from build123d import *

# Parameters (mm, degrees)
SKETCH1_R           = 1.1303
SKETCH1_W           = 3.2766
SKETCH1_H           = 18.2372
BOSS_EXTRUDE1_DEPTH = 1.5875
FILLET1_R           = 4.445
SKETCH2_W           = 81.9912
SKETCH2_H           = 2.0955
BOSS_EXTRUDE2_DEPTH = 3.175
SKETCH3_W           = 31.9024
SKETCH3_H           = 2.0955
CUT_EXTRUDE1_DEPTH  = 3.175


with BuildPart() as part:
    # Sketch1 → Boss-Extrude1 (new, symmetric)
    with BuildSketch(Plane(origin=(0, 0, 0), x_dir=(1, 0, 0), z_dir=(0, 1, 0))):
        Polygon((-38.5572, -41.9227), (-38.5572, 25.0825), (38.5572, 25.0825), (38.5572, -41.9227), (54.229, -41.9227), (54.229, 41.9227), (-54.229, 41.9227), (-54.229, -41.9227), align=None)
        with Locations(Location((-40.9956, -38.6969, 0), (0, 0, 270))):
            Circle(SKETCH1_R, mode=Mode.SUBTRACT)
        with Locations(Location((-40.9956, 22.3139, 0), (0, 0, 270))):
            Circle(SKETCH1_R, mode=Mode.SUBTRACT)
        with Locations(Location((40.9956, 22.3139, 0), (0, 0, 270))):
            Circle(SKETCH1_R, mode=Mode.SUBTRACT)
        with Locations(Location((40.9956, -38.6969, 0), (0, 0, 270))):
            Circle(SKETCH1_R, mode=Mode.SUBTRACT)
        with Locations((-50.5587, 10.0711)):
            Rectangle(SKETCH1_W, SKETCH1_H, mode=Mode.SUBTRACT)
        with Locations((-50.5587, -17.8689)):
            Rectangle(SKETCH1_W, SKETCH1_H, mode=Mode.SUBTRACT)
        with Locations((50.5587, -17.8689)):
            Rectangle(SKETCH1_W, SKETCH1_H, mode=Mode.SUBTRACT)
        with Locations((50.5587, 10.0711)):
            Rectangle(SKETCH1_W, SKETCH1_H, mode=Mode.SUBTRACT)
        Polygon((-20.5232, 36.6141), (-41.7322, 36.6141), (-41.7322, 39.8907), (-9.5758, 39.8907), (-9.5758, 37.2237), (-9.5758, 36.9697), (1.5748, 36.9697), (1.5748, 28.0289), (-20.5232, 28.0289), align=None, mode=Mode.SUBTRACT)
        Polygon((9.5758, 38.590972839), (9.5758, 39.8907), (39.5478, 39.8907), (39.5478, 37.1221), (44.5262, 37.1221), (44.5262, 30.7721), (35.7632, 30.7721), (35.7632, 36.6141), (9.5758, 36.6141), align=None, mode=Mode.SUBTRACT)
    extrude(amount=BOSS_EXTRUDE1_DEPTH, both=True)

    # Fillet1
    fillet1_edges = [part.edges().sort_by_distance(p)[0] for p in [
        (-54.229, 0, -41.9227),
        (54.229, 0, -41.9227),
        (54.229, 0, 41.9227),
        (-54.229, 0, 41.9227),
    ]]
    fillet(fillet1_edges, radius=FILLET1_R)

    # Sketch2 → Boss-Extrude2 (add)
    with BuildSketch(Plane(origin=(0, 1.5875, 0), x_dir=(1, 0, 0), z_dir=(0, 1, 0))):
        with Locations((0, -40.87495)):
            Rectangle(SKETCH2_W, SKETCH2_H)
    extrude(amount=-BOSS_EXTRUDE2_DEPTH)

    # Sketch3 → Cut-Extrude1 (cut)
    with BuildSketch(Plane(origin=(0, 1.5875, 0), x_dir=(1, 0, 0), z_dir=(0, 1, 0))):
        with Locations((-1.905, -40.87495)):
            Rectangle(SKETCH3_W, SKETCH3_H)
    extrude(amount=-CUT_EXTRUDE1_DEPTH, mode=Mode.SUBTRACT)


solid = part.part
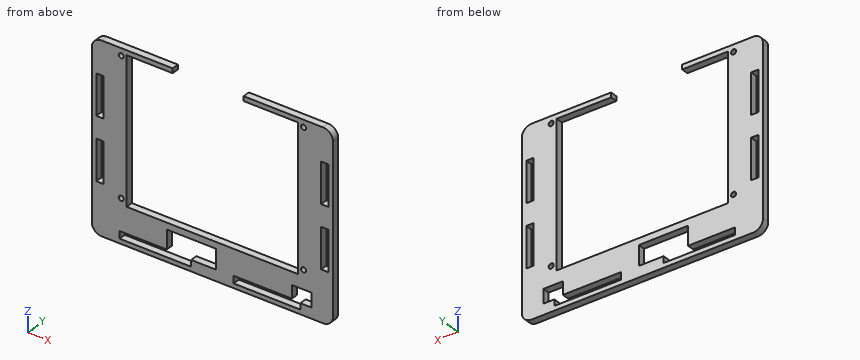
Source: CAD feature listing. Evaluate the final solid. Frame: model axes, mm. Round coordinates to 2 decimals unless told otherwise and drop trailing zeros. Loops run counter-clockwise (first coordinate to the right, second up) from the corner with the lowest first, then second, coordinate; pieces in that order, holes last.
Q1. Ray query, line 1 (X direction, y = 0.3, z = -31.5); line 2 (Z direction, x = -28.5, y = 0.3); line 3 (X direction, y = 1.1, z = -17.5). Return the intervals inside material, ascending.
Q2. First-contact query: P1, Ø1.4, axis at y = 0.5, z = -38.5, coming from the -X side; P2, Ø1.4, axis at x = 41, z = 38.7, coming from the -Y side; P3, Ø1, axis at y = 0.5, z = 41, coming from the +X side. Flat tips, straight axial feed; report the tip coordinate or a pass-through.
Q3. Section C-C, the plane x = 6.5. Return loops of the section in (y, z), plus the area to 3 significant figures.
Q4. Section D-D, the plane y = 0.8. State how many separate pieces and enclosed holes the cut face has, plus the area to 3 significant figures.
Q5. Section B-B, the plane x = -35.5. Return loops of the section in (y, z), plus the area to 3 significant figures.
Q6. Section A-A, the plane z = 4. Return loops of the section in (x, y), plus the area to 3 significant figures.
Solutions:
1. line 1: x = -54.23 to -20.52, 1.57 to 35.76, 44.53 to 54.23
1. line 2: z = -41.92 to -39.89, -36.61 to -25.08, 39.83 to 41.92
1. line 3: x = -54.23 to -52.2, -48.92 to -38.56, 38.56 to 48.92, 52.2 to 54.23
2. P1: stops at x = -54.22
2. P2: passes through
2. P3: stops at x = 53.04
3. outline: (-1.59, -41.92) - (1.59, -41.92) - (1.59, -25.08) - (-1.59, -25.08) - close
3. area: 53.5 mm2
4. separate pieces: 1
4. enclosed holes: 10
4. area: 3,300 mm2
5. outline: (-1.59, -41.92) - (1.59, -41.92) - (1.59, -39.89) - (-1.59, -39.89) - close; (-1.59, -36.61) - (1.59, -36.61) - (1.59, -25.08) - (-1.59, -25.08) - close; (-1.59, 39.83) - (1.59, 39.83) - (1.59, 41.92) - (-1.59, 41.92) - close
5. area: 49.7 mm2
6. outline: (-54.23, -1.59) - (-38.56, -1.59) - (-38.56, 1.59) - (-54.23, 1.59) - close; (38.56, -1.59) - (54.23, -1.59) - (54.23, 1.59) - (38.56, 1.59) - close
6. area: 99.5 mm2
